Geometry check sheet. Reference: the model listing, model coordinates, mm. Coordinates: 2 decimals unless noted, no trailing zeros. Write each loop counter-clockwise with the first axis right and the second up, starting at its lowest first coordinate (ties: lowest second). Pieces come first, ordered by that corner, then holes. Notation, with made-up numbers: (35.5, 73) -> (47.5, 73) arc R16 cw to (47.5, 86) -> close; hole circle Ø6 at (37.5, 3). An arc over 180 degrees is marked (long way). Answer in a Markdown table with one row per item. Add a question column.
Q1. Section check C-C, the plane x = 104.5. Record the boundary of the cut face in (y, z), and give its area (3 significant figures).
Q2. Section check A-A, the plane y = 3.4. Record the boundary of the cut face in (x, z).
Q3. Gauge pin test, flat end, axial feed: P1, Ø1, axis at x = 61.5, z = -82.5, coming from the +Y side. Record the tip position at first contact, or that the pin passes through.
Q4. Section check B-B, the plane z = -55.5. Record the boundary of the cut face in (x, y).
Q5. Thickness scan on line 1 (Y direction, x = -14.5, z = -141.5); line 2 (X direction, y = 3.2, z = -102.5); line 3 (X direction, y = 2.7, z = -103). Record the ranges inside material, lowest first.
```python
from build123d import *

# Parameters (mm, degrees)
SKETCH1_W           = 187
SKETCH1_H           = 222
BOSS_EXTRUDE1_DEPTH = 1
SKETCH2_R           = 1.5
BOSS_EXTRUDE2_DEPTH = 3


with BuildPart() as part:
    # Sketch1 → Boss-Extrude1 (new body)
    with BuildSketch(Plane(origin=(0, 0, 0), x_dir=(1, 0, 0), z_dir=(0, 1, 0))):
        with Locations((37.397058758, 75.462578399)):
            Rectangle(SKETCH1_W, SKETCH1_H)
    extrude(amount=BOSS_EXTRUDE1_DEPTH)

    # Sketch2 → Boss-Extrude2 (add)
    with BuildSketch(Plane(origin=(0, 1, 0), x_dir=(1, 0, 0), z_dir=(0, 1, 0))):
        with Locations((121.897058758, 165.632578399)):
            Circle(SKETCH2_R)
        with Locations((-37.614941242, 165.632578399)):
            Circle(SKETCH2_R)
        with Locations((121.897058758, 103.656578399)):
            Circle(SKETCH2_R)
        with Locations((-37.614941242, 103.652578399)):
            Circle(SKETCH2_R)
    extrude(amount=BOSS_EXTRUDE2_DEPTH)


solid = part.part
```
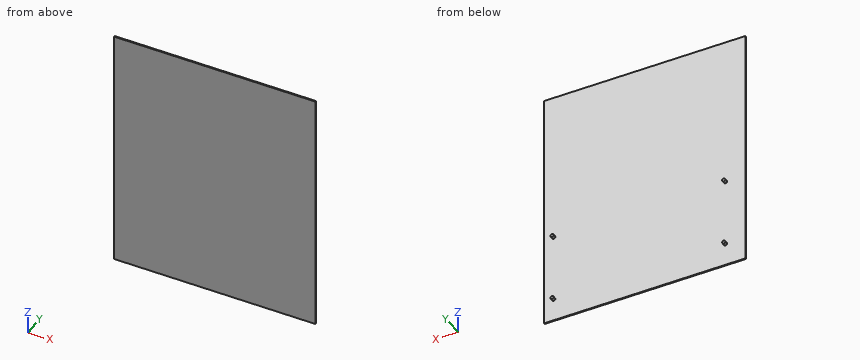
Calculated:
| question | item | result |
|---|---|---|
| 1 | outline | (0, -186.46) -> (1, -186.46) -> (1, 35.54) -> (0, 35.54) -> close |
| 1 | area | 222 mm² |
| 2 | outline | circle Ø3 at (-37.61, -165.63); circle Ø3 at (-37.61, -103.65); circle Ø3 at (121.9, -165.63); circle Ø3 at (121.9, -103.66) |
| 3 | P1 | stops at y = 1 |
| 4 | outline | (-56.1, 0) -> (130.9, 0) -> (130.9, 1) -> (-56.1, 1) -> close |
| 5 | line 1 | y = 0 to 1 |
| 5 | line 2 | x = -38.57 to -36.65, 120.94 to 122.85 |
| 5 | line 3 | x = -38.97 to -36.26, 120.55 to 123.25 |
